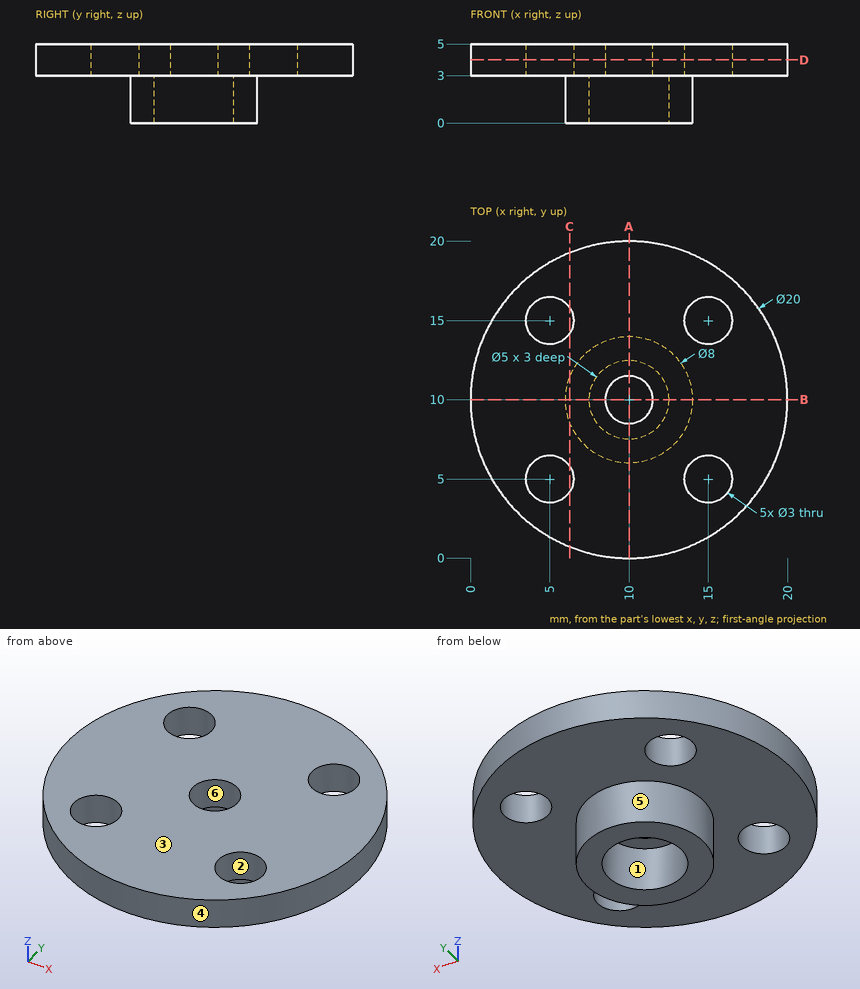
Print and shaded views of the part. All mm, measured from the part's lowest x, y and z. A direction names the side the tool comes from. Coordinates: 2 decimals unless noted, no trailing zeros. Order: outer loops, then holes, each group sorted by start corner. A loop starts at its lowest first (then second) coordinate and runs counter-clockwise, first axis right, second up. Notation, with made-up numbers: M 53,61.25 L 61,61.25 A20 ccw 61,68.25 Z; hole C -27,57 d2. An arc over 180 degrees is marked long. Answer as CSV lines item,"result".
1) Drill centre lines: L1, parallel to Y at x = 5, z = 3.9; L2, parallel to Y at x = 10, z = 2.45; L3, parallel to Z at x = 6.25, y = 13.25. Where is each one in solid material? Low to high. Write a range as from..to.
Verdict:
L1,"1.34..3.5, 6.5..13.5, 16.5..18.66"
L2,"6..7.5, 12.5..14"
L3,"3..5"
2) Cut at A-A (x = 10). List the corners of the cut face in (y, z), then the cut area to 3 significant figures.
Verdict:
outline,"M 0,3 L 6,3 L 6,0 L 7.5,0 L 7.5,3 L 8.5,3 L 8.5,5 L 0,5 Z; M 11.5,3 L 12.5,3 L 12.5,0 L 14,0 L 14,3 L 20,3 L 20,5 L 11.5,5 Z"
area,"43.0 mm2"
3) Flat gauge pins, fed straight in: P1, Ø1, axis at y = 10.5, z = 2, coming from the -X side; P2, Ø4, axis at x = 5, y = 15, coming from the -Z side; P3, Ø10, axis at x = 10.5, y = 13, coming from the -Z side; P4, Ø1.5, axis at x = 14.5, z = 3, coming from the -Y side. Where does each tip first touch, or does it go through?
Verdict:
P1,"x = 6"
P2,"z = 3"
P3,"z = 0"
P4,"y = 0.73"
4) Cut at C-C (x = 6.25). List the corners of the cut face in (y, z).
Verdict:
outline,"M 0.73,3 L 4.17,3 L 4.17,5 L 0.73,5 Z; M 5.83,3 L 8.61,3 L 8.61,0 L 11.39,0 L 11.39,3 L 14.17,3 L 14.17,5 L 5.83,5 Z; M 15.83,3 L 19.27,3 L 19.27,5 L 15.83,5 Z"
5) Mould opens along Y. For the marked faces 1, 2, 3 and 4 say: released by +Y, released by -Y, zero draft, split by the parting line, or undercut.
Verdict:
face 1,"undercut"
face 2,"undercut"
face 3,"zero draft"
face 4,"split by the parting line"
6) 3-axis set-ups, long thin cutter, end or side, ignore diameter. For the marked faces 5 and 6: which of +Z, -Z, +X, -X, +Y, -Y reach the whole face in a straight line?
Verdict:
face 5,"-Z"
face 6,"+Z, -Z"
7) Cut at D-D (z = 4). List the corners of the cut face in (x, y), then the cut area to 3 significant figures.
Verdict:
outline,"C 10,10 d20; hole C 5,5 d3; hole C 5,15 d3; hole C 10,10 d3; hole C 15,5 d3; hole C 15,15 d3"
area,"279 mm2"
